Source: CAD feature listing. Evaluate the final solid. Frame: model axes, mm. Face numbers are marked on the shaded views. A direction names the side the tool comes from. Give positions to 0.01 mm unless a question says otherwise; leave off trailing zeros. Write each loop counter-clockwise with the first axis right and the second up, starting at its lowest first coordinate (ties: lowest second). Pieces come first, ordered by that corner, then holes. Notation, with made-up numbers: (5, 69) -> (13, 69) arc R24 ccw to (13, 91) -> close; hole circle Ø11 at (45, -3.75). An arc over 180 degrees is marked (long way). Use a Markdown table: item, result. Add a question column.
```python
from build123d import *

# Parameters (mm, degrees)
SKETCH1_R                = 87
BOSS_EXTRUDE3_DEPTH      = 100
SKETCH2_R                = 45
BOSS_EXTRUDE4_DEPTH      = 20.5
SKETCH3_R                = 75
BOSS_EXTRUDE5_DEPTH      = 20
FILLET1_R                = 10
BOSS_EXTRUDE6_START      = 20.5
SKETCH4_R                = 45
BOSS_EXTRUDE6_DEPTH      = 20.5
BOSS_EXTRUDE7_START      = 20
SKETCH5_R                = 75
BOSS_EXTRUDE7_DEPTH      = 20
FILLET2_R                = 10
BOSS_EXTRUDE8_REACH      = 241.969
BOSS_EXTRUDE8_END_RADIUS = 87
SKETCH6_W                = 100
SKETCH6_H                = 141
SKETCH9_R                = 45
BOSS_EXTRUDE10_DEPTH     = 141
CUT_EXTRUDE2_DEPTH       = 374.425025993
CUT_EXTRUDE2_DEPTH_BACK  = 374.425025993
SKETCH21_W               = 216.769628827
SKETCH21_H               = 100


with BuildPart() as part:
    # Sketch1 → Boss-Extrude3 (new body)
    with BuildSketch(Plane(origin=(0, 0, 0), x_dir=(0, 0, -1), z_dir=(1, 0, 0))):
        Circle(SKETCH1_R)
    extrude(amount=BOSS_EXTRUDE3_DEPTH)

    # Sketch2 → Boss-Extrude4 (add)
    with BuildSketch(Plane(origin=(100, 0, 0), x_dir=(0, 0, -1), z_dir=(1, 0, 0))):
        Circle(SKETCH2_R)
    extrude(amount=BOSS_EXTRUDE4_DEPTH)

    # Sketch3 → Boss-Extrude5 (add)
    with BuildSketch(Plane(origin=(120.5, 0, 0), x_dir=(0, 0, -1), z_dir=(1, 0, 0))):
        Circle(SKETCH3_R)
    extrude(amount=BOSS_EXTRUDE5_DEPTH)

    # Fillet1
    fillet1_edges = [part.edges().sort_by_distance(p)[0] for p in [
        (140.5, 0, 75),
        (120.5, 0, 75),
    ]]
    fillet(fillet1_edges, radius=FILLET1_R - 0.0001)  # a hair under: the kernel refuses the full size

    # Sketch4 → Boss-Extrude6 (add)
    with BuildSketch(Plane.ZY.offset(BOSS_EXTRUDE6_START)):
        with Locations(Location((0, 0, 0), (0, 0, 180))):
            Circle(SKETCH4_R)
    extrude(amount=-BOSS_EXTRUDE6_DEPTH)

    # Sketch5 → Boss-Extrude7 (add)
    with BuildSketch(Plane.ZY.offset(20.5).offset(BOSS_EXTRUDE7_START)):
        Circle(SKETCH5_R)
    extrude(amount=-BOSS_EXTRUDE7_DEPTH)

    # Fillet2
    fillet2_edges = [part.edges().sort_by_distance(p)[0] for p in [
        (-20.5, 0, -75),
        (-40.5, 0, -75),
    ]]
    fillet(fillet2_edges, radius=FILLET2_R - 0.0001)  # a hair under: the kernel refuses the full size

    # Boss-Extrude8: up to this cylinder (the profile starts outside it)
    boss_extrude8_end = Plane(origin=(50, 0, 0), z_dir=(-1, 0, 0)) * Cylinder(BOSS_EXTRUDE8_END_RADIUS, 658.938, mode=Mode.PRIVATE)
    # Sketch6 → Boss-Extrude8 (add, up to the surface)
    with BuildSketch(Plane(origin=(0, 87, 0), x_dir=(1, 0, 0), z_dir=(0, 1, 0)), mode=Mode.PRIVATE) as boss_extrude8_sk1:
        with Locations((50, 0)):
            Rectangle(SKETCH6_W, SKETCH6_H)
    boss_extrude8_tool1 = extrude(boss_extrude8_sk1.sketch, amount=-BOSS_EXTRUDE8_REACH, mode=Mode.PRIVATE) - boss_extrude8_end
    add(boss_extrude8_tool1.solids().sort_by_distance((50, 87, 0))[0])
    add(boss_extrude8_tool1.solids().sort_by_distance((50, 87, 0))[1])

    # Sketch9 → Boss-Extrude10 (add)
    with BuildSketch(Plane(origin=(0, 0, -70.5), x_dir=(-1, 0, 0), z_dir=(0, 0, -1))):
        with BuildLine():
            Line((-100, 87), (0, 87))
            Line((0, 87), (0, 152.803089955))
            ThreePointArc((0, 152.803089955), (-50, 311), (-100, 152.803089955))
            Line((-100, 152.803089955), (-100, 87))
        make_face()
        with Locations((-50, 224)):
            Circle(SKETCH9_R, mode=Mode.SUBTRACT)
    extrude(amount=-BOSS_EXTRUDE10_DEPTH)

    # Sketch21 → Cut-Extrude2 (cut, two sides: drawn at the far end of the back side and taken through both)
    with BuildSketch(Plane(origin=(147, 0, 0), x_dir=(0, 1, 0), z_dir=(-1, 0, 0)).offset(-CUT_EXTRUDE2_DEPTH_BACK)):
        with Locations((227.184814414, 0)):
            Rectangle(SKETCH21_W, SKETCH21_H)
    extrude(amount=CUT_EXTRUDE2_DEPTH + CUT_EXTRUDE2_DEPTH_BACK, mode=Mode.SUBTRACT)


solid = part.part
```
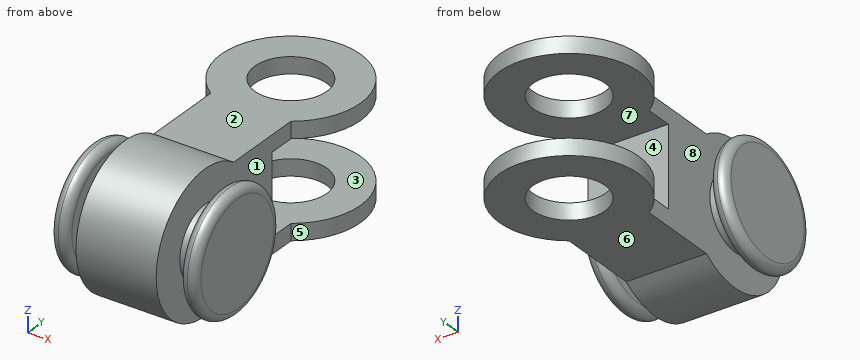
(1) Cut plane D-D on y = 224. Return the cut outline in (x, z), then the cut area to 3 significant figures.
(2) Material intervals for L1, parallel to X at y = -58.5, z = 15.5; L2, parallel to X at y = 46.5, z = -51.5; L3, parallel to Z at x = 88.5, y = 133, sorted ascending.
(3) Access query for the marked faces 5, 6, 7 and 8. Directions: +Z, -Z, +X, -X, +Y, -Y. A direction counts if a zero-diameter tool reaches every point of the face in a straight line with its end or side. Return the directions, or none.
(4) Mould query, pull axis Z, two halves, no side actions, for the marked faces 1, 2, 3 and 4. Classes: +Z half, -Z half, draft (parallel to the pull), parting line (faces both ways), or undercut.
(5) Cut plane A-A on y = 123.5. Return the cut outline in (x, z).
(6) First-contact query: pin 1 Ø1 at (x, z) = (22.5, -11) entering from -Y; pin 2 Ø10 at (x, z) = (105.5, -37.5) entering from +Y; pin 3 Ø5 at (x, z) = (42.5, -33) entering from +Y. Flat tips, straight axial feed; report the tip coordinate or a pass-through.
(7) Cut plane C-C on x = -15. Return the cut outline in (y, z).
Output:
| question | item | result |
|---|---|---|
| 1 | outline | (-37, -70.5) -> (5, -70.5) -> (5, -50) -> (-37, -50) -> close; (-37, 50) -> (5, 50) -> (5, 70.5) -> (-37, 70.5) -> close; (95, -70.5) -> (137, -70.5) -> (137, -50) -> (95, -50) -> close; (95, 50) -> (137, 50) -> (137, 70.5) -> (95, 70.5) -> close |
| 1 | area | 3,440 mm^2 |
| 2 | L1 | -40.5 to -20.5, 0 to 100, 120.5 to 140.5 |
| 2 | L2 | -39.49 to -21.51, 0 to 100, 121.51 to 139.49 |
| 2 | L3 | -70.5 to -50, 50 to 70.5 |
| 3 | face 5 | +Z, -Z |
| 3 | face 6 | -Z, +X, -X, +Y |
| 3 | face 7 | +X, -X, +Y |
| 3 | face 8 | none |
| 4 | face 1 | draft |
| 4 | face 2 | +Z half |
| 4 | face 3 | undercut |
| 4 | face 4 | undercut |
| 5 | outline | (0, -70.5) -> (100, -70.5) -> (100, -50) -> (0, -50) -> close; (0, 50) -> (100, 50) -> (100, 70.5) -> (0, 70.5) -> close |
| 6 | pin 1 | y = -86.36 |
| 6 | pin 2 | y = 31.12 |
| 6 | pin 3 | y = 118.8 |
| 7 | outline | circle Ø90 at (0, 0); (166.17, -70.5) -> (281.83, -70.5) -> (281.83, -50) -> (166.17, -50) -> close; (166.17, 50) -> (281.83, 50) -> (281.83, 70.5) -> (166.17, 70.5) -> close |
